Geometry: final body of the model. Coordinates: model frame, mm. Coordinates: 2 decimals unless noted, no trailing zeros. Loops run counter-clockwise (first coordinate to the right, second up) from the corner with the lowest first, then second, coordinate; pieces in that order, holes last. Notation, with made-up numbers: (2.5, -6) - (34.5, -6) arc R19 ccw to (34.5, 23) - close; hole circle Ø8 at (87, -23). An arc over 180 degrees is marked (long way). Put each result on its own line as item: value. Start each with the question number.
1) Section C-C on y = -25. Output: boundary loops of the cut face in (x, z) (3 decimals).
2) Section B-B on x = 0. Output: boundary loops of the cut face in (y, z) (3 decimals), and give its area (3 significant figures).
3) Material intervals for line 1 along Z through (x, y) = (0, -41) (3 decimals); line 2 along Z through (x, y) = (-7.5, -12.7); line 3 along X through (y, z) = (-32, 1), sorted ascending. Write a range as from..to.
4) Contact query for flat-ended pins moving along their axis: pin 1 Ø3 at (y, z) = (-8.5, 2.5) entering from +X; pin 2 Ø4 at (x, z) = (0, 0) entering from +Y; pin 3 Ø1 at (y, z) = (-40.5, -2) entering from +X; pin 4 Ø1 at (x, y) = (-3, -25.5) entering from -Z. Output: stop coordinate, or through.
5) Draft query along X for faces 1 (the cylindrical face through (9.085, -38.365, 2.861)), 2 (the cylindrical face through (-3.03, -39.41, -0.95)), 3 (the flat face through (3.4, 0, 0.1)). Return one class per face: +X half, -X half, draft (parallel to the pull), parting line (faces both ways), or undercut.
6) Section A-A on y = -12. Output: boundary loops of the cut face in (x, z) (3 decimals).
```python
from build123d import *

# Parameters (mm, degrees)
F0_R     = 9.525
F1_DEPTH = 77.7748
F3_D     = 6.35
F3_DEPTH = 77.72908
F3_TIP   = 1.9077324654
F4_SIZE2 = 1.5748
F4_SIZE  = 1.5748
F6_D     = 4.7498
F6_DEPTH = 19.05
F6_TIP   = 1.4269838841
F8_D     = 4.7498
F8_DEPTH = 19.05
F8_START = 3.1750001
F8_TIP   = 1.4269838841


with BuildPart() as f1:
    # F0 (on Front) → F1 (new body)
    with BuildSketch(Plane.XZ):
        Circle(F0_R)
    extrude(amount=F1_DEPTH)

    # F3
    with Locations(Plane(origin=(0, 0, 0), x_dir=(1, 0, 0), z_dir=(0, 1, 0))):
        with Locations((0, 0)):
            Hole(F3_D / 2, depth=F3_DEPTH)
            with Locations((0, 0, -(F3_DEPTH + F3_TIP / 2))):  # 118° drill point
                Cone(0, F3_D / 2, F3_TIP, mode=Mode.SUBTRACT)

    # F4
    f4_edges = [f1.edges().sort_by_distance(p)[0] for p in [
        (-9.525, -77.7748, 0),
        (-9.525, 0, 0),
    ]]
    chamfer(f4_edges, length=F4_SIZE, length2=F4_SIZE2)

    # F6 (one way)
    with BuildSketch(Plane.YZ):
        with Locations((-12.7, 0)):
            Circle(F6_D / 2)
    extrude(amount=-F6_DEPTH, mode=Mode.SUBTRACT)
    with Locations(Plane.YZ):
        with Locations((-12.7, 0)):
            with Locations((0, 0, -(F6_DEPTH + F6_TIP / 2))):  # 118° drill point
                Cone(0, F6_D / 2, F6_TIP, mode=Mode.SUBTRACT)

    # F8
    # its depths count from where the whole tool has entered the part; down to there all is cleared
    with Locations(Plane(origin=(0, 0, 0), x_dir=(0, 1, 0), z_dir=(-1, 0, 0)).offset(-F8_START)):
        with Locations((-12.7, 0)):
            Hole(F8_D / 2, depth=F8_DEPTH)
            with Locations((0, 0, -(F8_DEPTH + F8_TIP / 2))):  # 118° drill point
                Cone(0, F8_D / 2, F8_TIP, mode=Mode.SUBTRACT)


solid = f1.part
```
Answer block:
1. outline: circle Ø19.05 at (0, 0); hole circle Ø6.35 at (0, 0)
2. outline: (-77.775, -7.95) - (-76.2, -9.525) - (-1.575, -9.525) - (0, -7.95) - (0, -3.175) - (-77.729, -3.175) - (-77.775, -3.099) - close; (-77.775, 3.099) - (-77.729, 3.175) - (0, 3.175) - (0, 7.95) - (-1.575, 9.525) - (-76.2, 9.525) - (-77.775, 7.95) - close
2. area: 983 mm²
3. line 1: z = -9.525..-3.175, 3.175..9.525
3. line 2: z = -5.87..-2.37, 2.37..5.87
3. line 3: x = -9.47..-3.01, 3.01..9.47
4. pin 1: stops at x = 9.47
4. pin 2: passes through
4. pin 3: stops at x = 9.41
4. pin 4: stops at z = -9.19
5. face 1: parting line
5. face 2: undercut
5. face 3: draft
6. outline: (-9.251, -2.269) arc R9.525 ccw to (9.251, -2.269) - (2.22, -2.269) arc R3.175 cw to (-2.22, -2.269) - close; (-9.251, 2.269) - (-2.22, 2.269) arc R3.175 cw to (2.22, 2.269) - (9.251, 2.269) arc R9.525 ccw to start
